Verification items for the finished model (mm, model axes). Give positions to 0.01 mm unless a question says otherwise; leave off trailing zeros. Loops run counter-clockwise (first coordinate to the right, second up) from the corner with the lowest first, then second, coordinate; pieces in that order, holes last. Notation, with made-up numbers: (75, 39.25) - (83, 39.25) arc R24 ccw to (83, 51.25) - close; hole circle Ø11 at (-30.75, -7). An arc over 180 degrees is marked (long way). One line per item, written item: value. Start each with the question number.
1. Gauge pin test, flat ends, axial feed: pin 1 (3 mm diameter, centred on y = 280.5, z = 72.5, fed in from +X); pin 2 (4 mm diameter, centred on x = 304.5, z = -76, fed in from -Y); pin 3 (2 mm diameter, centred on y = 81, z = -1.5, fed in from -X). Record the tip position at first contact, or that the pin passes through.
2. Sectioned sample at C-C (z = 65.5). Count the separate pieces of the cut face and the enclosed holes in it, plus the area to 3 significant figures.
3. Sectioned sample at D-D (x = -438). Record the cut outline in (y, z), plus the area to 3 significant figures.
4. Mould release check, pull along Y, two halves, no side actions. Record for faces 1 (the flat face through (-146, -321, 0)), 2 (the cylindrical face through (173.458, 379.418, 44.37)), 3 (the cylindrical face through (332.884, -104.83, 99.86)): pulls with the +Y half, pulls with the -Y half, needs draft (parallel to the pull), parting line crosses it, or undercut.
5. Sectioned sample at A-A (x = 0). Record the cut outline in (y, z).
6. Scan lines: L1, parallel to Y at x = 169.5, z = 81.5; L2, parallel to Y at x = 331.5, z = 55.5; L3, parallel to Y at x = -334, z = 56. Record each from-to range of solid material in increasing order. Write a range as [from, to].
Autodesk Inventor part; units mm, degrees
ref_plane "YZ Plane" through (0, 0, 0) normal (1, 0, 0) x (0, 1, 0)
ref_plane "XZ Plane" through (0, 0, 0) normal (0, 1, 0) x (-1, 0, 0)
ref_plane "XY Plane" through (0, 0, 0) normal (0, 0, 1) x (1, 0, 0)
sketch "Schizzo1" plane through (0, 0, 0) normal (0, 0, 1) x (1, 0, 0)
  circle A0 centre (0, 0) radius 485.5
  circle A1 centre (0, 0) radius 325
  circle A2 centre (0, 0) radius 334
  circle A3 centre (0, 0) radius 349
  circle A4 centre (0, 0) radius 438 construction
  circle A5 centre (0, 438) radius 22.5
  circle A6 centre (-97.4642, 427.0184) radius 22.5
  circle A7 centre (-190.0411, 394.6244) radius 22.5
  circle A8 centre (-273.0885, 342.4422) radius 22.5
  circle A9 centre (-342.4422, 273.0885) radius 22.5
  circle A10 centre (-394.6244, 190.0411) radius 22.5
  circle A11 centre (-427.0184, 97.4642) radius 22.5
  circle A12 centre (-438, 0) radius 22.5
  circle A13 centre (-427.0184, -97.4642) radius 22.5
  circle A14 centre (-394.6244, -190.0411) radius 22.5
  circle A15 centre (-342.4422, -273.0885) radius 22.5
  circle A16 centre (-273.0885, -342.4422) radius 22.5
  circle A17 centre (-190.0411, -394.6244) radius 22.5
  circle A18 centre (-97.4642, -427.0184) radius 22.5
  circle A19 centre (0, -438) radius 22.5
  circle A20 centre (97.4642, -427.0184) radius 22.5
  circle A21 centre (190.0411, -394.6244) radius 22.5
  circle A22 centre (273.0885, -342.4422) radius 22.5
  circle A23 centre (342.4422, -273.0885) radius 22.5
  circle A24 centre (394.6244, -190.0411) radius 22.5
  circle A25 centre (427.0184, -97.4642) radius 22.5
  circle A26 centre (438, 0) radius 22.5
  circle A27 centre (427.0184, 97.4642) radius 22.5
  circle A28 centre (394.6244, 190.0411) radius 22.5
  circle A29 centre (342.4422, 273.0885) radius 22.5
  circle A30 centre (273.0885, 342.4422) radius 22.5
  circle A31 centre (190.0411, 394.6244) radius 22.5
  circle A32 centre (97.4642, 427.0184) radius 22.5
  dimension "d5" = 876
  dimension "d0" = 971
  dimension "d1" = 650
  dimension "d2" = 668
  dimension "d3" = 698
  dimension "d6" = 45
  dimension "d9" = 360
extrude "Estrusione1" add sketch "Schizzo1" along normal blind 90 contours A0
extrude "Estrusione2" add sketch "Schizzo1" along normal blind 110 and the other way blind 105 contours A2 | A3
fillet "Raccordo1" radius 2 1 edges at (-349, 0, -105)
properties part number "messa in tavola"
Results are:
1. pin 1: stops at x = 397.33
1. pin 2: stops at y = -174.05
1. pin 3: stops at x = -339.71
2. separate pieces: 1
2. enclosed holes: 29
2. area: 364,000 mm^2
3. outline: (-209.44, 0) - (-117.1, 0) - (-117.1, 90) - (-209.44, 90) - close; (-77.83, 0) - (-22.5, 0) - (-22.5, 90) - (-77.83, 90) - close; (22.5, 0) - (77.83, 0) - (77.83, 90) - (22.5, 90) - close; (117.1, 0) - (209.44, 0) - (209.44, 90) - (117.1, 90) - close
3. area: 26,600 mm^2
4. face 1: needs draft
4. face 2: undercut
4. face 3: parting line crosses it
5. outline: (-485.5, 0) - (-460.5, 0) - (-460.5, 90) - (-485.5, 90) - close; (-415.5, 0) - (-349, 0) - (-349, -103) arc R2 ccw to (-347, -105) - (-325, -105) - (-325, 110) - (-349, 110) - (-349, 90) - (-415.5, 90) - close; (325, -105) - (347, -105) arc R2 ccw to (349, -103) - (349, 0) - (415.5, 0) - (415.5, 90) - (349, 90) - (349, 110) - (325, 110) - close; (460.5, 0) - (485.5, 0) - (485.5, 90) - (460.5, 90) - close
6. L1: y = [-454.95, -403.81], [-385.44, -277.3], [277.3, 385.44], [403.81, 454.95]
6. L2: y = [-354.71, -292.75], [-253.43, 253.43], [292.75, 354.71]
6. L3: y = [-352.36, -293.94], [-252.23, 252.23], [293.94, 352.36]
